Model file for the job. Use its own axes, mm. A direction names the side the tool comes from. Coordinates: 2 decimals unless noted, no trailing zeros. Loops run counter-clockwise (first coordinate to the right, second up) from the corner with the lowest first, then second, coordinate; pieces in that order, holes last.
Autodesk Inventor part; units mm, degrees
ref_plane "Plano de trabalho1" through (0, 10, 0) normal (0, 1, 0) x (1, 0, 0)
ref_plane "YZ Plane" through (0, 0, 0) normal (1, 0, 0) x (0, 1, 0)
ref_plane "XZ Plane" through (0, 0, 0) normal (0, 1, 0) x (-1, 0, 0)
sketch "Esboço1" plane through (0, 0, 0) normal (0, 1, 0) x (-1, 0, 0)
  circle A0 centre (0, 0) radius 0.75
  dimension "d1" = 1.5
extrude "Extrusão1" add sketch "Esboço1" along normal blind 9.6
ref_plane "Plano de trabalho1" through (0, 10, 0) normal (0, 1, 0) x (1, 0, 0)
sketch "Esboço2" plane through (0, 10, 0) normal (0, 1, 0) x (1, 0, 0)
  circle A0 centre (0, 0) radius 1.25
  dimension "d5" = 2.5
loft "Transição1" add profiles "Esboço2" section 1 edges at (0.75, 9.6, 0)
sketch "Esboço3" plane through (0, 10, 0) normal (0, 1, 0) x (1, 0, 0)
  line L0 (0.25, -0.875) -> (-0.25, -0.875)
  line L1 (-0.25, -0.875) -> (-0.25, 0.875)
  line L2 (-0.25, 0.875) -> (0.25, 0.875)
  line L3 (0.25, 0.875) -> (0.25, -0.875)
  line L4 (0.25, -0.875) -> (-0.25, 0.875) construction
  line L5 (-0.25, -0.875) -> (0.25, 0.875) construction
  line L6 (-0.875, -0.25) -> (0.875, -0.25)
  line L7 (0.875, -0.25) -> (0.875, 0.25)
  line L8 (0.875, 0.25) -> (-0.875, 0.25)
  line L9 (-0.875, 0.25) -> (-0.875, -0.25)
  line L10 (-0.875, -0.25) -> (0.875, 0.25) construction
  line L11 (0.875, -0.25) -> (-0.875, 0.25) construction
  point P0 (0, 0)
  point P1 (-0.25, 0.25)
  point P2 (-0.25, -0.25)
  point P3 (0.25, -0.25)
  point P4 (0.25, 0.25)
  dimension "d10" = 0.5
  dimension "d11" = 1.75
  dimension "d14" = 1.75
  dimension "d15" = 0.5
extrude "Extrusão2" cut sketch "Esboço3" against normal blind 0.25
thread "Rosca1"
properties part number "Parafuso"
Q1. Flat gauge pins, fed straight in: P1, Ø1, axis at x = -0.5, y = 7, coming from the +Z side; P2, Ø1, axis at y = 7, z = 1, coming from the -X side. Where does each tip first touch, or does it go through?
Answers:
P1: stops at z = 0.75
P2: stops at x = -0.56
Q2. Drill centre lines: line 1 (Z direction, x = -0.05, y = 4.75); line 2 (Y direction, x = 0.15, z = 0.05); line 3 (X direction, y = 7.5, z = -0.15). Where is each one in solid material? Low to high.
Answers:
line 1: z = -0.75 to 0.75
line 2: y = 0 to 9.75
line 3: x = -0.73 to 0.73
Q3. Which spindle directions (+Z, -Z, +X, -X, +Y, -Y) get a long thin tool onto all of the face, cutting with end or side? Do faces 1 (the cylindrical face through (0.75, 4.73, -0.03)), 2 (the flat face through (0, 0, 0)). Say none if no direction does.
Answers:
face 1: -Y
face 2: +Z, -Z, +X, -X, -Y
Q4. Slice it at B-B (y = 7.5). List the corners of the cut face in (x, z).
Answers:
outline: circle Ø1.5 at (0, 0)
Q5. Slice it at A-A (x = 0). List the corners of the cut face in (y, z) (3 decimals), and give its area (3 significant figures).
Answers:
outline: (0, -0.75) - (9.6, -0.75) - (10, -1.25) - (10, -0.875) - (9.75, -0.875) - (9.75, 0.875) - (10, 0.875) - (10, 1.25) - (9.6, 0.75) - (0, 0.75) - close
area: 14.8 mm2
